Build history of the part. All positions in model axes, mm. Face numbers are marked on the shaded views. A direction names the side the tool comes from. Round coordinates to 2 decimals unless told otherwise and drop trailing zeros. Write each loop counter-clockwise with the first axis right and the second up, starting at its lowest first coordinate (ties: lowest second). Pieces come first, ordered by that corner, then holes. Notation, with made-up numbers: M 39.5,16 L 62.5,16 A9 cw 62.5,32 Z; hole C -33,-35 d9. An arc over 180 degrees is marked long. Use a Markdown table: item, result.
from build123d import *

# Parameters (mm, degrees)
EXTRUDE_1_DEPTH     = 40
SKETCH_2_R          = 1.6
CUT_EXTRUDE_1_DEPTH = 40


with BuildPart() as part:
    # 草图1 → 凸台-拉伸1 (new body)
    with BuildSketch(Plane.XY):
        with BuildLine():
            Line((-14.465476141, 1), (-10.307764064, 1))
            ThreePointArc((-10.307764064, 1), (-9.671555054, 1.22848325), (-9.326072248, 1.80952381))
            ThreePointArc((-9.326072248, 1.80952381), (0, 9.5), (9.326072248, 1.80952381))
            ThreePointArc((9.326072248, 1.80952381), (9.671555054, 1.22848325), (10.307764064, 1))
            Line((10.307764064, 1), (14.465476141, 1))
            Line((14.465476141, 1), (20, 1))
            ThreePointArc((20, 1), (20.707106781, 1.292893219), (21, 2))
            Line((21, 2), (21, 5))
            ThreePointArc((21, 5), (20.707106781, 5.707106781), (20, 6))
            Line((20, 6), (13.829316686, 6))
            ThreePointArc((13.829316686, 6), (13.305681748, 6.148057249), (12.937102706, 6.548387097))
            ThreePointArc((12.937102706, 6.548387097), (0, 14.5), (-12.937102706, 6.548387097))
            ThreePointArc((-12.937102706, 6.548387097), (-13.305681748, 6.148057249), (-13.829316686, 6))
            Line((-13.829316686, 6), (-20, 6))
            ThreePointArc((-20, 6), (-20.707106781, 5.707106781), (-21, 5))
            Line((-21, 5), (-21, 2))
            ThreePointArc((-21, 2), (-20.707106781, 1.292893219), (-20, 1))
            Line((-20, 1), (-14.465476141, 1))
        make_face()
    extrude(amount=EXTRUDE_1_DEPTH)

    # 草图2 → 切除-拉伸1 (cut)
    with BuildSketch(Plane(origin=(0, 6, 0), x_dir=(1, 0, 0), z_dir=(0, 1, 0))):
        with Locations(Location((-17, -8, 0), (0, 0, 270))):
            Circle(SKETCH_2_R)
        with Locations(Location((17, -8, 0), (0, 0, 270))):
            Circle(SKETCH_2_R)
        with Locations(Location((17, -32, 0), (0, 0, 270))):
            Circle(SKETCH_2_R)
        with Locations(Location((-17, -32, 0), (0, 0, 270))):
            Circle(SKETCH_2_R)
    extrude(amount=-CUT_EXTRUDE_1_DEPTH, mode=Mode.SUBTRACT)


solid = part.part
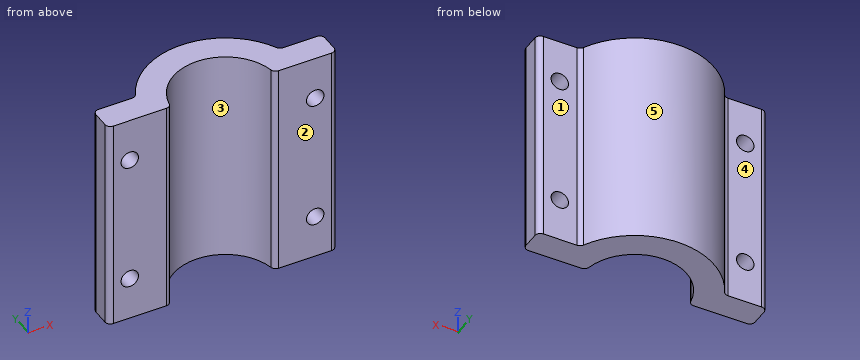
Q1. Cut at D-D on z = 18. Give the cut face in (x, y).
Response values:
| item | result |
|---|---|
| outline | M -21,2 A1 ccw -20,1 L -10.31,1 A1 ccw -9.33,1.81 A9.5 cw 9.33,1.81 A1 ccw 10.31,1 L 20,1 A1 ccw 21,2 L 21,5 A1 ccw 20,6 L 13.83,6 A1 cw 12.94,6.55 A14.5 ccw -12.94,6.55 A1 cw -13.83,6 L -20,6 A1 ccw -21,5 Z |
Q2. Cut at A-A on z = 8. Give the cut face in (x, y).
Response values:
| item | result |
|---|---|
| outline | M -21,2 A1 ccw -20,1 L -18.6,1 L -18.6,6 L -20,6 A1 ccw -21,5 Z; M -15.4,1 L -10.31,1 A1 ccw -9.33,1.81 A9.5 cw 9.33,1.81 A1 ccw 10.31,1 L 15.4,1 L 15.4,6 L 13.83,6 A1 cw 12.94,6.55 A14.5 ccw -12.94,6.55 A1 cw -13.83,6 L -15.4,6 Z; M 18.6,1 L 20,1 A1 ccw 21,2 L 21,5 A1 ccw 20,6 L 18.6,6 Z |
Q3. Which spindle directions (+Z, -Z, +X, -X, +Y, -Y) get a long thin tool onto all of the face, cutting with end or side? Do the marked faces 1 and 2. Say none if no direction does.
Response values:
| item | result |
|---|---|
| face 1 | +Z, -Z, +X, +Y |
| face 2 | +Z, -Z, +X, -X, -Y |
Q4. Cut at B-B on x = -17. Give the cut face in (y, z).
Response values:
| item | result |
|---|---|
| outline | M 1,0 L 6,0 L 6,6.4 L 1,6.4 Z; M 1,9.6 L 6,9.6 L 6,30.4 L 1,30.4 Z; M 1,33.6 L 6,33.6 L 6,40 L 1,40 Z |
Q5. Two-plate mould, pull along X, no slides. Class the marked faces 3, 4 and 5: +X half, -X half, draft (parallel to the pull), parting line (faces both ways), or undercut.
Response values:
| item | result |
|---|---|
| face 3 | undercut |
| face 4 | draft |
| face 5 | parting line |
Q6. Cut at C-C on y = 7.25. Give the cut face in (x, z), and give its area (3 significant figures).
Response values:
| item | result |
|---|---|
| outline | M -12.56,0 L -6.14,0 L -6.14,40 L -12.56,40 Z; M 6.14,0 L 12.56,0 L 12.56,40 L 6.14,40 Z |
| area | 513 mm2 |
Q7. Drop flat-ended pins along their axis: P1, Ø5, axis at x = -17, z = 8, coming from the +Y side; P2, Ø7, axis at x = 17, z = 11.5, coming from the +Y side; P3, Ø8, axis at x = -0.5, z = 16, coming from the -Y side. Give the stop position or say it passes through.
Response values:
| item | result |
|---|---|
| P1 | stops at y = 6 |
| P2 | stops at y = 6.06 |
| P3 | stops at y = 8.37 |
Q8. Drill centre lines: L1, parallel to X at y = 2.45, z = 8; L2, parallel to X at y = 2.95, z = 32; L3, parallel to X at y = 6.5, z = 4. Where is each one in solid material? Low to high.
Response values:
| item | result |
|---|---|
| L1 | x = -21 to -18.6, -15.4 to -9.18, 9.18 to 15.4, 18.6 to 21 |
| L2 | x = -21 to -18.6, -15.4 to -9.03, 9.03 to 15.4, 18.6 to 21 |
| L3 | x = -12.96 to -6.93, 6.93 to 12.96 |
